Verification items for the finished model (mm, model axes). Coordinates: 2 decimals unless noted, no trailing zeros. Write each loop counter-clockwise with the first axis right and the second up, starting at its lowest first coordinate (ties: lowest second). Pieces come first, ordered by that corner, then holes. Notation, with made-up numbers: (6, 54) - (55, 54) arc R25 ccw to (55, 79) - close; hole circle Ø7 at (12, -4). An arc over 180 degrees is marked (long way). Use one line per item in the form item = value. Start each with the question number.
(1) Sectioned sample at A-A (x = -74). Record the cut outline in (y, z).
(2) Gauge pin test, flat ends, axial feed: pin 1 Ø3.5 at (x, z) = (11, -9) entering from +Y; pin 2 Ø2.5 at (x, z) = (-45, -46) entering from -Y; pin 3 Ø1 at (y, z) = (1.5, -31) entering from -X. Record the tip position at first contact, or that the pin passes through.
(3) Material ranges on line 1 (X direction, y = 1.4, z = 17.5); line 2 (Z direction, x = 4.5, y = 0.45); line 3 (X direction, y = 1.5, z = -34.5), recorded low to high. Write a range as [from, to].
(4) Mould release check, pull along Z, two halves, no side actions. Record for faces 1 (the flat face through (-80, 1, 0)), 2 (the cylindrical face through (20.18, 1.52, 30.37)), 3 (the cylindrical face through (-19.99, 1.48, 11.89)): released by +Z, released by -Z, zero draft, split by the parting line, or undercut.
(5) Sectioned sample at B-B (y = 0.7). Count the separate pieces of the cut face and the enclosed holes in it, and give its area (3 significant figures).
from build123d import *

# Parameters (mm, degrees)
SKETCH_1_R      = 1.5
SKETCH_1_R_2    = 13
SKETCH_1_W      = 15
SKETCH_1_H      = 15
EXTRUDE_1_DEPTH = 3
FILLET_1_R      = 2.5
FILLET_2_R      = 5


with BuildPart() as part:
    # 草图1 → 凸台-拉伸1 (new body)
    with BuildSketch(Plane(origin=(0, 0, 0), x_dir=(1, 0, 0), z_dir=(0, 1, 0))):
        Polygon((-60, 50), (0, 50), (20, 30), (25, 30), (25, -30), (20, -30), (0, -50), (-60, -50), (-80, -30), (-80, 30), align=None)
        with Locations(Location((-45, 46, 0), (0, 0, 270))):
            Circle(SKETCH_1_R, mode=Mode.SUBTRACT)
        with Locations(Location((0, 29, 0), (0, 0, 90))):
            Circle(SKETCH_1_R_2, mode=Mode.SUBTRACT)
        with Locations(Location((-25, 46, 0), (0, 0, 270))):
            Circle(SKETCH_1_R, mode=Mode.SUBTRACT)
        with Locations(Location((-45, -46, 0), (0, 0, 90))):
            Circle(SKETCH_1_R, mode=Mode.SUBTRACT)
        with Locations(Location((-25, -46, 0), (0, 0, 90))):
            Circle(SKETCH_1_R, mode=Mode.SUBTRACT)
        with Locations(Location((-60, 35.75, 0), (0, 0, 270))):
            Circle(SKETCH_1_R, mode=Mode.SUBTRACT)
        with Locations(Location((-32, 35.75, 0), (0, 0, 270))):
            Circle(SKETCH_1_R, mode=Mode.SUBTRACT)
        with Locations(Location((-60, -35.75, 0), (0, 0, 270))):
            Circle(SKETCH_1_R, mode=Mode.SUBTRACT)
        with Locations(Location((-26, -32, 0), (0, 0, 270))):
            Circle(SKETCH_1_R, mode=Mode.SUBTRACT)
        with Locations(Location((-44, -32, 0), (0, 0, 270))):
            Circle(SKETCH_1_R, mode=Mode.SUBTRACT)
        with Locations(Location((11, -9, 0), (0, 0, 270))):
            Circle(SKETCH_1_R, mode=Mode.SUBTRACT)
        with Locations(Location((11, 9, 0), (0, 0, 270))):
            Circle(SKETCH_1_R, mode=Mode.SUBTRACT)
        with Locations(Location((-21, -13, 0), (0, 0, 270))):
            Circle(SKETCH_1_R, mode=Mode.SUBTRACT)
        with Locations(Location((0, -46, 0), (0, 0, 270))):
            Circle(SKETCH_1_R, mode=Mode.SUBTRACT)
        with Locations(Location((0, 46, 0), (0, 0, 270))):
            Circle(SKETCH_1_R, mode=Mode.SUBTRACT)
        with Locations(Location((0, -29, 0), (0, 0, 270))):
            Circle(SKETCH_1_R_2, mode=Mode.SUBTRACT)
        with Locations(Location((22, 9, 0), (0, 0, 270))):
            Circle(SKETCH_1_R, mode=Mode.SUBTRACT)
        with Locations(Location((22, -9, 0), (0, 0, 270))):
            Circle(SKETCH_1_R, mode=Mode.SUBTRACT)
        with Locations(Location((21, 25, 0), (0, 0, 270))):
            Circle(SKETCH_1_R, mode=Mode.SUBTRACT)
        with Locations(Location((21, -25, 0), (0, 0, 270))):
            Circle(SKETCH_1_R, mode=Mode.SUBTRACT)
        with Locations(Location((0, -12, 0), (0, 0, 270))):
            Circle(SKETCH_1_R, mode=Mode.SUBTRACT)
        with Locations(Location((0, 12, 0), (0, 0, 90))):
            Circle(SKETCH_1_R, mode=Mode.SUBTRACT)
        with BuildLine():
            Line((-76, -25), (-76, 25))
            ThreePointArc((-76, 25), (-74, 27), (-72, 25))
            Line((-72, 25), (-72, -25))
            ThreePointArc((-72, -25), (-74, -27), (-76, -25))
        make_face(mode=Mode.SUBTRACT)
        with BuildLine():
            Line((-66, -8), (-49.165832492, -8))
            ThreePointArc((-49.165832492, -8), (-48.371424783, -5.849344075), (-47.437917706, -3.755312305))
            Line((-47.437917706, -3.755312305), (-66, 6.961510904))
            Line((-66, 6.961510904), (-66, -8))
        make_face(mode=Mode.SUBTRACT)
        Polygon((-61, 30.75), (-48.272965565, 30.75), (-66, 13.351215514), (-66, 25.75), align=None, mode=Mode.SUBTRACT)
        with BuildLine():
            Line((-21, 30.75), (-21, 15.588862316))
            ThreePointArc((-21, 15.588862316), (-26.243676334, 14.407879152), (-31.244687695, 12.437917706))
            Line((-31.244687695, 12.437917706), (-41.817173337, 30.75))
            Line((-41.817173337, 30.75), (-21, 30.75))
        make_face(mode=Mode.SUBTRACT)
        with BuildLine():
            Line((-61.900970054, 10.368437553), (-44.937917706, 0.574814714))
            ThreePointArc((-44.937917706, 0.574814714), (-40.703188492, 5.703188492), (-35.574814714, 9.937917706))
            Line((-35.574814714, 9.937917706), (-45.25562103, 26.705566103))
            Line((-45.25562103, 26.705566103), (-61.900970054, 10.368437553))
        make_face(mode=Mode.SUBTRACT)
        with Locations((-58.5, -20.5)):
            Rectangle(SKETCH_1_W, SKETCH_1_H, mode=Mode.SUBTRACT)
        with BuildLine():
            ThreePointArc((-15.95445115, 9.95445115), (-36.460547805, 1.460547805), (-44.95445115, -19.04554885))
            ThreePointArc((-44.95445115, -19.04554885), (-42.95445115, -21.04554885), (-40.95445115, -19.04554885))
            ThreePointArc((-40.95445115, -19.04554885), (-33.63212068, -1.36787932), (-15.95445115, 5.95445115))
            ThreePointArc((-15.95445115, 5.95445115), (-13.95445115, 7.95445115), (-15.95445115, 9.95445115))
        make_face(mode=Mode.SUBTRACT)
    extrude(amount=EXTRUDE_1_DEPTH)

    # 圆角1
    fillet_1_edges = [part.edges().sort_by_distance(p)[0] for p in [
        (-66, 1.5, -6.961510904),
        (-66, 1.5, 8),
        (-49.165832492, 1.5, 8),
        (-47.437917706, 1.5, 3.755312305),
        (-61, 1.5, -30.75),
        (-66, 1.5, -25.75),
        (-66, 1.5, -13.351215514),
        (-48.272965565, 1.5, -30.75),
        (-45.25562103, 1.5, -26.705566103),
        (-61.900970054, 1.5, -10.368437553),
        (-44.937917706, 1.5, -0.574814714),
        (-35.574814714, 1.5, -9.937917706),
        (-66, 1.5, 13),
        (-66, 1.5, 28),
        (-51, 1.5, 28),
        (-51, 1.5, 13),
        (-31.244687695, 1.5, -12.437917706),
        (-21, 1.5, -15.588862316),
        (-21, 1.5, -30.75),
        (-41.817173337, 1.5, -30.75),
    ]]
    fillet(fillet_1_edges, radius=FILLET_1_R)

    # 圆角2
    fillet_2_edges = [part.edges().sort_by_distance(p)[0] for p in [
        (20, 1.5, -30),
        (20, 1.5, 30),
    ]]
    fillet(fillet_2_edges, radius=FILLET_2_R)


solid = part.part
Answers below:
q1.outline = (0, -36) - (3, -36) - (3, -27) - (0, -27) - close; (0, 27) - (3, 27) - (3, 36) - (0, 36) - close
q2.pin_1 = 3
q2.pin_2 = through
q2.pin_3 = -79.5
q3.line_1 = [-80, -76], [-72, -66], [-51, -44.91], [-40.91, -6.06], [6.06, 25]
q3.line_2 = [-45.5, -41.2], [-16.8, 16.8], [41.2, 45.5]
q3.line_3 = [-75.5, -60.83], [-59.17, -32.83], [-31.17, -11.78], [11.78, 15.5]
q4.face_1 = zero draft
q4.face_2 = released by +Z
q4.face_3 = undercut
q5.separate_pieces = 1
q5.enclosed_holes = 29
q5.area = 6,800 mm2
